Check sheet for the modelled part. Datum: model origin and axes. Units: mm. A direction names the side the tool comes from. Coordinates: 2 decimals unless noted, no trailing zeros. Loops run counter-clockwise (first coordinate to the right, second up) from the corner with the lowest first, then second, coordinate; pieces in that order, holes last.
from build123d import *

# Parameters (mm, degrees)
SKETCH1_W             = 100
SKETCH1_H             = 48
BOSS_EXTRUDE1_DEPTH   = 8
SKETCH2_W             = 46
SKETCH2_H             = 48
BOSS_EXTRUDE2_DEPTH   = 10
CUT_EXTRUDE1_DEPTH    = 72.61005516
FILLET1_R             = 8
M4_TAPPED_HOLE1_D     = 3.3
M4_TAPPED_HOLE1_DEPTH = 10
M4_TAPPED_HOLE1_TIP   = 0.991420021
M8_TAPPED_HOLE1_D     = 6.8


with BuildPart() as part:
    # Sketch1 → Boss-Extrude1 (new body)
    with BuildSketch(Plane(origin=(0, 0, 0), x_dir=(1, 0, 0), z_dir=(0, 1, 0))):
        Rectangle(SKETCH1_W, SKETCH1_H)
    extrude(amount=BOSS_EXTRUDE1_DEPTH)

    # Sketch2 → Boss-Extrude2 (add)
    with BuildSketch(Plane(origin=(0, 8, 0), x_dir=(1, 0, 0), z_dir=(0, 1, 0))):
        Rectangle(SKETCH2_W, SKETCH2_H)
    extrude(amount=BOSS_EXTRUDE2_DEPTH)

    # Sketch3 → Cut-Extrude1 (cut, through all)
    with BuildSketch(Plane.XY.offset(24)):
        with BuildLine():
            Line((-8, 13), (-8, 18))
            Line((-8, 18), (8, 18))
            Line((8, 18), (8, 13))
            ThreePointArc((8, 13), (0, 5), (-8, 13))
        make_face()
    extrude(amount=-CUT_EXTRUDE1_DEPTH, mode=Mode.SUBTRACT)

    # Fillet1
    fillet1_edges = [part.edges().sort_by_distance(p)[0] for p in [
        (50, 4, 24),
        (-50, 4, 24),
        (-50, 4, -24),
        (50, 4, -24),
    ]]
    fillet(fillet1_edges, radius=FILLET1_R)

    # M4 Tapped Hole1
    with Locations(Plane(origin=(0, 18, 0), x_dir=(1, 0, 0), z_dir=(0, 1, 0))):
        with Locations((-15, 14), (-15, -14), (15, -14), (15, 14)):
            Hole(M4_TAPPED_HOLE1_D / 2, depth=M4_TAPPED_HOLE1_DEPTH)
            with Locations((0, 0, -(M4_TAPPED_HOLE1_DEPTH + M4_TAPPED_HOLE1_TIP / 2))):  # 118° drill point
                Cone(0, M4_TAPPED_HOLE1_D / 2, M4_TAPPED_HOLE1_TIP, mode=Mode.SUBTRACT)

    # M8 Tapped Hole1 (through all)
    with Locations(Plane(origin=(0, 8, 0), x_dir=(1, 0, 0), z_dir=(0, 1, 0))):
        with Locations((-38, 12), (-38, -12), (38, -12), (38, 12)):
            Hole(M8_TAPPED_HOLE1_D / 2)


solid = part.part
(1) Section check A-A, the plane y = 15.5. Enter the section's corners in (x, z), plus the area to 3 significant figures.
(2) Section check C-C, the plane z = 0. Enter the section's corners in (x, y), plus the area to 3 significant figures.
(3) Section check D-D, the plane y = 11.5. Enter the section's corners in (x, z), plus the area to 3 significant figures.
(4) Section check B-B, the plane x = 38. Enter the section's corners in (y, z).
(5) Scan lines: line 1 along Z through (x, y) = (15, 15); line 2 along X through (y, z) = (3.25, -12); line 3 along Z through (x, y) = (-38, 3). Record each from-to range of solid material in increasing order.
(6) Set-up check for faces 4 (the face through (47.594, 4.056, -21.719)), 5 (the face through (-8, 15, 0)), 6 (the face through (-0.59, 4.87, 24)), 7 (the face through (13.476, 12.93, -13.368)), 8 (the face through (23, 13, 0)): record each of +Z, -Z, +X, -X, +Y, -Y from which the full face is reachable in a straight line by a thin tool's end or side.
(7) Gauge pin test, flat ends, axial feed: P1, Ø6, axis at y = 8.5, z = -7.5, coming from the +X side; P2, Ø3, axis at y = 12, z = 9, coming from the +X side; P3, Ø2, axis at x = -15, z = 14, coming from the +Y side; P4, Ø1, axis at y = 14, z = 7, coming from the -X side. Record the tip position at first contact, or that the pin passes through.
(8) Draft check along X on faces 1 (the face through (-15.04, 7.18, -14.28)), 2 (the face through (15, 18, 0)), 3 (the face through (-47.719, 4.056, -21.594)). Enter one of: pulls with the +X half, pulls with the -X half, needs draft (parallel to the pull), parting line crosses it, or undercut.
Determined:
1. outline: (-23, -24) - (-8, -24) - (-8, 24) - (-23, 24) - close; (8, -24) - (23, -24) - (23, 24) - (8, 24) - close; hole circle Ø3.3 at (-15, -14); hole circle Ø3.3 at (-15, 14); hole circle Ø3.3 at (15, -14); hole circle Ø3.3 at (15, 14)
1. area: 1,410 mm2
2. outline: (-50, 0) - (50, 0) - (50, 8) - (23, 8) - (23, 18) - (8, 18) - (8, 13) arc R8 cw to (-8, 13) - (-8, 18) - (-23, 18) - (-23, 8) - (-50, 8) - close
2. area: 1,080 mm2
3. outline: (-23, -24) - (-7.86, -24) - (-7.86, 24) - (-23, 24) - close; (7.86, -24) - (23, -24) - (23, 24) - (7.86, 24) - close; hole circle Ø3.3 at (-15, -14); hole circle Ø3.3 at (-15, 14); hole circle Ø3.3 at (15, -14); hole circle Ø3.3 at (15, 14)
3. area: 1,420 mm2
4. outline: (0, -24) - (8, -24) - (8, -15.4) - (0, -15.4) - close; (0, -8.6) - (8, -8.6) - (8, 8.6) - (0, 8.6) - close; (0, 15.4) - (8, 15.4) - (8, 24) - (0, 24) - close
5. line 1: z = -24 to -15.65, -12.35 to 12.35, 15.65 to 24
5. line 2: x = -50 to -41.4, -34.6 to 34.6, 41.4 to 50
5. line 3: z = -24 to -15.4, -8.6 to 8.6, 15.4 to 24
6. face 4: -Z, +X, +Y, -Y
6. face 5: +Z, -Z, +Y
6. face 6: +Z, +X, -X, +Y, -Y
6. face 7: +Y
6. face 8: +Z, -Z, +X, +Y
7. P1: stops at x = 50
7. P2: stops at x = 23
7. P3: stops at y = 7.61
7. P4: stops at x = -23
8. face 1: undercut
8. face 2: needs draft
8. face 3: pulls with the -X half
